from build123d import *

# Parameters (mm, degrees)
F2_R     = 152.4
F2_R_2   = 44.45
F3_DEPTH = 6.35
F4_DEPTH = 12.7


with BuildPart() as f1:
    # F0 (on Front) → F1 (revolve)
    with BuildSketch(Plane.XZ):
        Polygon((-114.3, 215.9), (-114.3, 228.6), (-152.4, 228.6), (-152.4, -228.6), (-114.3, -228.6), (-114.3, -215.9), (-139.7, -215.9), (-139.7, 215.9), align=None)
    revolve(axis=Axis((0, 0, 0), (0, 0, -1)))

    # F2 (on Top) → F3 (join, symmetric)
    with BuildSketch(Plane.XY):
        Circle(F2_R)
        Circle(F2_R_2, mode=Mode.SUBTRACT)
    extrude(amount=F3_DEPTH, both=True)

    # F2 (on Top) → F4 (join, symmetric)
    with BuildSketch(Plane.XY):
        Circle(F2_R)
        Circle(F2_R_2, mode=Mode.SUBTRACT)
    extrude(amount=F4_DEPTH, both=True)


solid = f1.part
Work out the finished part from the listing and answer in its coordinate system (mm). A direction names the side the tool comes from. Coordinates: 2 decimals unless noted, no trailing zeros. Write each loop counter-clockwise with the first axis right and the second up, starting at its lowest first coordinate (ties: lowest second). Pieces come first, ordered by that corner, then holes. Notation, with made-up numbers: M 32,1.25 L 40,1.25 A19 ccw 40,36.25 Z; hole C 56.25,77 d1. An arc over 180 degrees is marked long. Answer as CSV lines item,"result". Start each with the question number.
Item 1: Section D-D on y = 76 is taken. Write down the section's boundary in (x, z).
Item 2: A tool of negligible diameter and unlimited length cuts with its end or side. For faces 4 (the face through (114.5, 0.7, 215.9)), 5 (the face through (114.19, 5.03, 222.34)), 6 (the face through (42.397, 13.352, -0.178)), from which of +Z, -Z, +X, -X, +Y, -Y can it reach the whole face along a straight path? Write none if from no direction.
Item 3: Flat-ended cylindrical pins translate along their axes: P1, Ø8, axis at x = 115, z = -62.5, coming from the -Y side; P2, Ø10, axis at y = 98.5, z = 40, coming from the -X side; P3, Ø1, axis at x = 5, y = -78.5, coming from the +Z side. Find the tip coordinate at first contact, or state that the pin passes through.
Item 4: Consider L1, parallel to Z at x = -120, y = -10; L2, parallel to Y at x = 0, z = -116.5; L3, parallel to Y at x = 0, z = -219. Determine where each line is inside the solid, lowest interval first.
Item 5: Determine the mould class of faces 1 (the face through (110.86, -85.01, 115.72)), 2 (the face through (114.19, 5.03, -222.16)), 3 (the face through (-22, 114, -228.6)) for opening direction Z: released by +Z, released by -Z, zero draft, split by the parting line, or undercut.
Item 6: Section C-C on z = -60.5 is taken. Write down the section's boundary in (x, y).
Item 7: Section A-A on x = 0 is taken. Write down the section's boundary in (y, z), and give its area (3 significant figures).
Checks:
1,outline,"M -132.1,-228.6 L -85.37,-228.6 L -85.37,-215.9 L -117.22,-215.9 L -117.22,-12.7 L 117.22,-12.7 L 117.22,-215.9 L 85.37,-215.9 L 85.37,-228.6 L 132.1,-228.6 L 132.1,228.6 L 85.37,228.6 L 85.37,215.9 L 117.22,215.9 L 117.22,12.7 L -117.22,12.7 L -117.22,215.9 L -85.37,215.9 L -85.37,228.6 L -132.1,228.6 Z"
2,face 4,"none"
2,face 5,"+Z"
2,face 6,"+Z, -Z"
3,P1,"stops at y = -104.43"
3,P2,"stops at x = -120.35"
3,P3,"stops at z = 12.7"
4,L1,"z = -228.6 to -215.9, -12.7 to 12.7, 215.9 to 228.6"
4,L2,"y = -152.4 to -139.7, 139.7 to 152.4"
4,L3,"y = -152.4 to -114.3, 114.3 to 152.4"
5,face 1,"undercut"
5,face 2,"zero draft"
5,face 3,"released by -Z"
6,outline,"C 0,0 d304.8; hole C 0,0 d279.4"
7,outline,"M -152.4,-228.6 L -114.3,-228.6 L -114.3,-215.9 L -139.7,-215.9 L -139.7,-12.7 L -44.45,-12.7 L -44.45,12.7 L -139.7,12.7 L -139.7,215.9 L -114.3,215.9 L -114.3,228.6 L -152.4,228.6 Z; M 44.45,-12.7 L 139.7,-12.7 L 139.7,-215.9 L 114.3,-215.9 L 114.3,-228.6 L 152.4,-228.6 L 152.4,228.6 L 114.3,228.6 L 114.3,215.9 L 139.7,215.9 L 139.7,12.7 L 44.45,12.7 Z"
7,area,"17,700 mm²"
